Check sheet for the modelled part. Datum: model origin and axes. Units: mm. A direction names the side the tool comes from. Give positions to 0.01 mm unless a question says otherwise; leave off trailing zeros. Write each loop counter-clockwise with the first axis right and the second up, starting at its lowest first coordinate (ties: lowest second). Pieces come first, ordered by that corner, then holes. Notation, with made-up numbers: M 57,42 L 80,42 A8 cw 80,46 Z; hole C -27.75,56.5 d10. An arc over 180 degrees is marked long. Write item = value, one per line. Start each with the question number.
1) Set-up check for faces 5 (the face through (41, 2, -62)), 6 (the face through (-62, 2, -40)), 7 (the face through (62, 6, 0)): record each of +Z, -Z, +X, -X, +Y, -Y from which the full face is reachable in a straight line by a thin tool's end or side.
2) Sectioned sample at A-A, the plane z = -43. Record the cut outline in (x, y).
3) Sectioned sample at D-D, the plane z = 20. Record the cut outline in (x, y), then the cut area to 3 significant figures.
4) Gauge pin test, flat ends, axial feed: pin 1 (5 mm diameter, centred on x = 39, z = -8, fed in from +Y); pin 2 (1.6 mm diameter, centred on x = 63.5, y = 2.5, fed in from -Z); pin 3 (2.5 mm diameter, centred on y = 2, z = 35.5, fed in from +X). Record the tip position at first contact, or that the pin passes through.
5) Draft check along X on faces 1 (the face through (0, 4, 64)), 2 (the face through (38.1, 1.5, -30.8)), 3 (the face through (24.51, 1.48, -41.89)), 4 (the face through (-62, 2, 40)). Enter one of: pulls with the +X half, pulls with the -X half, needs draft (parallel to the pull), parting line crosses it, or undercut.
6) Sectioned sample at C-C, the plane y = 6.5. Record the cut outline in (x, z).
7) Sectioned sample at B-B, the plane x = -39. Record the cut outline in (y, z).
8) Scan lines: L1, parallel to X at y = 1.15, z = -32; L2, parallel to X at y = 1.7, z = 23; L3, parallel to X at y = 7.75, z = -15. Record each from-to range of solid material in increasing order.
from build123d import *

# Parameters (mm, degrees)
SKETCH_1_W          = 128
SKETCH_1_H          = 128
EXTRUDE_1_DEPTH     = 8
CUT_EXTRUDE_1_DEPTH = 8
SKETCH_3_W          = 124
SKETCH_3_H          = 124
CUT_EXTRUDE_2_DEPTH = 5
FILLET_1_R          = 5
FILLET_2_R          = 5
FILLET_3_R          = 5
FILLET_4_R          = 5
SKETCH_4_R          = 1.5
CUT_EXTRUDE_3_DEPTH = 4


with BuildPart() as part:
    # 草图1 → 凸台-拉伸1 (new body)
    with BuildSketch(Plane(origin=(0, 0, 0), x_dir=(1, 0, 0), z_dir=(0, 1, 0))):
        Rectangle(SKETCH_1_W, SKETCH_1_H)
    extrude(amount=EXTRUDE_1_DEPTH)

    # 草图2 → 切除-拉伸1 (cut)
    with BuildSketch(Plane(origin=(0, 8, 0), x_dir=(1, 0, 0), z_dir=(0, 1, 0))):
        Polygon((-64, 64), (-64, 24), (-62, 24), (-62, 62), (-24, 62), (-24, 64), align=None)
        Polygon((-64, -24), (-62, -24), (-62, -62), (-24, -62), (-24, -64), (-64, -64), align=None)
        Polygon((24, -62), (24, -64), (64, -64), (64, -24), (62, -24), (62, -62), align=None)
        Polygon((64, 24), (62, 24), (62, 62), (24, 62), (24, 64), (64, 64), align=None)
    extrude(amount=-CUT_EXTRUDE_1_DEPTH, mode=Mode.SUBTRACT)

    # 草图3 → 切除-拉伸2 (cut)
    with BuildSketch(Plane(origin=(0, 8, 0), x_dir=(1, 0, 0), z_dir=(0, 1, 0))):
        Rectangle(SKETCH_3_W, SKETCH_3_H)
    extrude(amount=-CUT_EXTRUDE_2_DEPTH, mode=Mode.SUBTRACT)

    # 圆角1
    fillet_1_edges = [part.edges().sort_by_distance(p)[0] for p in [
        (-62, 1.5, 62),
    ]]
    fillet(fillet_1_edges, radius=FILLET_1_R)

    # 圆角2
    fillet_2_edges = [part.edges().sort_by_distance(p)[0] for p in [
        (62, 1.5, 62),
    ]]
    fillet(fillet_2_edges, radius=FILLET_2_R)

    # 圆角3
    fillet_3_edges = [part.edges().sort_by_distance(p)[0] for p in [
        (62, 1.5, -62),
    ]]
    fillet(fillet_3_edges, radius=FILLET_3_R)

    # 圆角4
    fillet_4_edges = [part.edges().sort_by_distance(p)[0] for p in [
        (-62, 1.5, -62),
    ]]
    fillet(fillet_4_edges, radius=FILLET_4_R)

    # 草图4 → 切除-拉伸3 (cut)
    with BuildSketch(Plane.XZ):
        with Locations(Location((-23.5, -43, 0), (0, 0, 270))):
            Circle(SKETCH_4_R)
        with Locations(Location((23.5, -43, 0), (0, 0, 270))):
            Circle(SKETCH_4_R)
        with Locations(Location((-23.5, 23, 0), (0, 0, 270))):
            Circle(SKETCH_4_R)
        with Locations(Location((23.5, 23, 0), (0, 0, 270))):
            Circle(SKETCH_4_R)
        with Locations(Location((-39, -32, 0), (0, 0, 270))):
            Circle(SKETCH_4_R)
        with Locations(Location((39, -32, 0), (0, 0, 270))):
            Circle(SKETCH_4_R)
        with Locations(Location((-39, -8, 0), (0, 0, 270))):
            Circle(SKETCH_4_R)
        with Locations(Location((39, -8, 0), (0, 0, 270))):
            Circle(SKETCH_4_R)
    extrude(amount=-CUT_EXTRUDE_3_DEPTH, mode=Mode.SUBTRACT)


solid = part.part
Data:
q1.face_5 = -Z, +X, +Y, -Y
q1.face_6 = -Z, -X, +Y, -Y
q1.face_7 = +Z, -Z, +Y
q2.outline = M -62,0 L -25,0 L -25,3 L -62,3 Z; M -22,0 L 22,0 L 22,3 L -22,3 Z; M 25,0 L 62,0 L 62,3 L 25,3 Z
q3.outline = M -64,0 L 64,0 L 64,8 L 62,8 L 62,3 L -62,3 L -62,8 L -64,8 Z
q3.area = 404 mm2
q4.pin_1 = 3
q4.pin_2 = -24
q4.pin_3 = 62
q5.face_1 = needs draft
q5.face_2 = undercut
q5.face_3 = undercut
q5.face_4 = pulls with the -X half
q6.outline = M -64,-24 L -62,-24 L -62,24 L -64,24 Z; M -24,-64 L 24,-64 L 24,-62 L -24,-62 Z; M -24,62 L 24,62 L 24,64 L -24,64 Z; M 62,-24 L 64,-24 L 64,24 L 62,24 Z
q7.outline = M 0,-62 L 3,-62 L 3,-33.5 L 0,-33.5 Z; M 0,-30.5 L 3,-30.5 L 3,-9.5 L 0,-9.5 Z; M 0,-6.5 L 3,-6.5 L 3,62 L 0,62 Z
q8.L1 = -62 to -40.5, -37.5 to 37.5, 40.5 to 62
q8.L2 = -64 to -25, -22 to 22, 25 to 64
q8.L3 = -64 to -62, 62 to 64
